```python
from build123d import *

# Parameters (mm, degrees)
BOSS_EXTRUDE1_DEPTH     = 5
BOSS_EXTRUDE2_DEPTH     = 27.5
BOSS_EXTRUDE3_DEPTH     = 10
CUT_EXTRUDE2_DEPTH      = 51.717354111
CUT_EXTRUDE2_DEPTH_BACK = 51.717354111
SKETCH5_3_W             = 6.5
SKETCH5_3_H             = 2
SKETCH5_3_W_2           = 20
BOSS_EXTRUDE4_DEPTH     = 2.75
CUT_EXTRUDE3_DEPTH      = 54.359629019
CUT_EXTRUDE3_DEPTH_BACK = 24
M4_CLEARANCE_HOLE1_D    = 4.5


with BuildPart() as part:
    # Sketch1 → Boss-Extrude1 (new body)
    with BuildSketch(Plane(origin=(0, 0, 0), x_dir=(1, 0, 0), z_dir=(0, 1, 0))):
        with BuildLine():
            Line((-36.5, 15), (36.5, 15))
            ThreePointArc((36.5, 15), (40.035533906, 13.535533906), (41.5, 10))
            Line((41.5, 10), (41.5, -10))
            ThreePointArc((41.5, -10), (40.035533906, -13.535533906), (36.5, -15))
            Line((36.5, -15), (-36.5, -15))
            ThreePointArc((-36.5, -15), (-40.035533906, -13.535533906), (-41.5, -10))
            Line((-41.5, -10), (-41.5, 10))
            ThreePointArc((-41.5, 10), (-40.035533906, 13.535533906), (-36.5, 15))
        make_face()
        with BuildLine():
            Line((-31.5, 7.5), (-31.5, -7.5))
            ThreePointArc((-31.5, -7.5), (-34.5, -10.5), (-37.5, -7.5))
            Line((-37.5, -7.5), (-37.5, 7.5))
            ThreePointArc((-37.5, 7.5), (-34.5, 10.5), (-31.5, 7.5))
        make_face(mode=Mode.SUBTRACT)
        with BuildLine():
            Line((31.5, 7.5), (31.5, -7.5))
            ThreePointArc((31.5, -7.5), (34.5, -10.5), (37.5, -7.5))
            Line((37.5, -7.5), (37.5, 7.5))
            ThreePointArc((37.5, 7.5), (34.5, 10.5), (31.5, 7.5))
        make_face(mode=Mode.SUBTRACT)
    extrude(amount=-BOSS_EXTRUDE1_DEPTH)

    # Sketch2 → Boss-Extrude2 (add, symmetric)
    with BuildSketch(Plane(origin=(0, 0, 0), x_dir=(0, 0, -1), z_dir=(1, 0, 0))):
        with BuildLine():
            Line((-15, 0), (0, 0))
            Line((0, 0), (0, 18))
            Line((0, 18), (-2.75, 18))
            add(Edge.make_bspline(
                [(-15, 0), (-3.342305564, 4.287493928), (-2.75, 18)],
                knots=[0, 0, 0, 1, 1, 1], degree=2))
        make_face()
        with BuildLine():
            Line((0, 18), (0, 0))
            Line((0, 0), (15, 0))
            add(Edge.make_bspline(
                [(15, 0), (3.342305564, 4.287493928), (2.75, 18)],
                knots=[0, 0, 0, 1, 1, 1], degree=2))
            Line((2.75, 18), (0, 18))
        make_face()
    extrude(amount=BOSS_EXTRUDE2_DEPTH, both=True)

    # Sketch2<3> → Boss-Extrude3 (add, symmetric)
    with BuildSketch(Plane(origin=(0, 0, 0), x_dir=(0, 0, -1), z_dir=(1, 0, 0))):
        with BuildLine():
            Line((-15, 0), (-15, 25))
            Line((-15, 25), (-8, 25))
            Line((-8, 25), (-2.75, 23))
            Line((-2.75, 23), (-2.75, 18))
            add(Edge.make_bspline(
                [(-15, 0), (-3.342305564, 4.287493928), (-2.75, 18)],
                knots=[0, 0, 0, 1, 1, 1], degree=2))
        make_face()
        with BuildLine():
            add(Edge.make_bspline(
                [(15, 0), (3.342305564, 4.287493928), (2.75, 18)],
                knots=[0, 0, 0, 1, 1, 1], degree=2))
            Line((2.75, 18), (2.75, 23))
            Line((2.75, 23), (8, 25))
            Line((8, 25), (15, 25))
            Line((15, 25), (15, 0))
        make_face()
    extrude(amount=BOSS_EXTRUDE3_DEPTH, both=True)

    # Sketch5 → Cut-Extrude2 (cut, two sides: drawn at the far end of the back side and taken through both)
    with BuildSketch(Plane.XY.offset(-CUT_EXTRUDE2_DEPTH_BACK)):
        Polygon((-27.5, 18), (-27.5, 0), (-21.5, 18), align=None)
        Polygon((21.5, 18), (27.5, 0), (27.5, 18), align=None)
    extrude(amount=CUT_EXTRUDE2_DEPTH + CUT_EXTRUDE2_DEPTH_BACK, mode=Mode.SUBTRACT)

    # Sketch5<3> → Boss-Extrude4 (add, symmetric)
    with BuildSketch(Plane.XY):
        with Locations((13.25, 19)):
            Rectangle(SKETCH5_3_W, SKETCH5_3_H)
        with Locations((-13.25, 19)):
            Rectangle(SKETCH5_3_W, SKETCH5_3_H)
        with Locations((0, 19)):
            Rectangle(SKETCH5_3_W_2, SKETCH5_3_H)
    extrude(amount=BOSS_EXTRUDE4_DEPTH, both=True)

    # Sketch6 → Cut-Extrude3 (cut, two sides: drawn at the far end of the back side and taken through both)
    with BuildSketch(Plane.XZ.offset(5).offset(-CUT_EXTRUDE3_DEPTH_BACK)):
        Polygon((16, 2.25), (10, 2.25), (-10, 2.25), (-16, 2.25), (-16, -2.25), (-10, -2.25), (10, -2.25), (16, -2.25), align=None)
    extrude(amount=CUT_EXTRUDE3_DEPTH + CUT_EXTRUDE3_DEPTH_BACK, mode=Mode.SUBTRACT)

    # M4 Clearance Hole1 (through all)
    with Locations(Plane(origin=(0, 20, 0), x_dir=(1, 0, 0), z_dir=(0, 1, 0))):
        with Locations((0, 0)):
            Hole(M4_CLEARANCE_HOLE1_D / 2)


solid = part.part
```
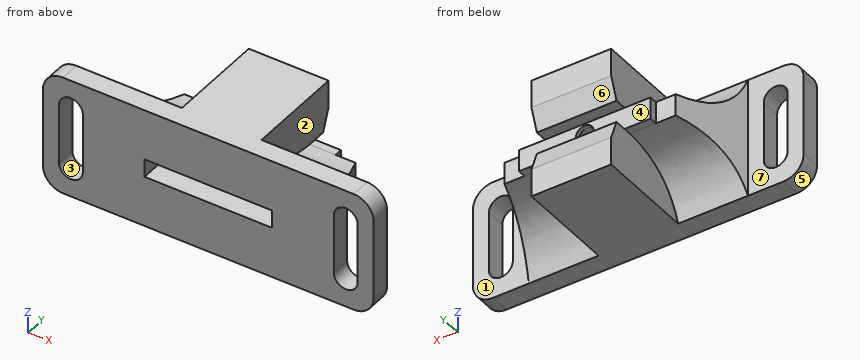
For this review, take the finished solid that the model builds, in its own axes (mm). Face numbers are marked on the shaded views. A direction names the side the tool comes from. Coordinates: 2 decimals unless noted, no trailing zeros. Write each loop counter-clockwise with the first axis right and the second up, starting at its lowest first coordinate (ties: lowest second). Pieces come first, ordered by that corner, then holes. Notation, with made-up numbers: (16, -36.75) - (26, -36.75) arc R29 cw to (26, -11.75) - close; hole circle Ø4 at (3, 49). An arc over 180 degrees is marked (long way). Answer in a Markdown table with one row per item. Add a question column.
Q1. We need section C-C, the plane z = 6.5. Count the separate pieces of the cut face and the enclosed holes in it, and give its area (3 significant figures).
Q2. We need section B-B, the plane z = 0. State the section outline as (x, y) points, and give its area (4 significant figures).
Q3. Draft analysis for pull direction Z (two halves, no side actions). For the marked faces 5, 6 and 7, state which applies: +Z half, -Z half, draft (parallel to the pull), parting line (faces both ways), or undercut.
Q4. Tool access review of the marked faces 1, 2, 3 and 4: name each direction out of +Z, -Z, +X, -X, +Y, -Y from which nothing blocks a thin tool from reaching the whole face with its end or side.
Q5. For P1, Ø1, axis at y = 17, z = -2, coming from the -X side; P2, Ø4, axis at x = 36.5, z = -2.5, coming from the +Y side; P3, Ø1, axis at y = 4.5, z = 11, coming from the -X side, all flat-tipped, find the tip position at first contact; note any pin that passes through.
Q6. We need section A-A, the plane x = -34.5. State the section outline as (y, z) points.
Q7. For probe 1 along X at (y, z) = (-1, 0); probe 2 along Z at (x, y) = (0, 19.45); probe 3 along Z at (x, y) = (-0.5, 22.5), list the stretches that pass through material, from the lowest coordinate up.
Answer list:
| question | item | result |
|---|---|---|
| 1 | separate pieces | 3 |
| 1 | enclosed holes | 0 |
| 1 | area | 1,040 mm2 |
| 2 | outline | (-41.5, -5) - (-37.5, -5) - (-37.5, 0) - (-41.5, 0) - close; (-31.5, -5) - (-16, -5) - (-16, 19) - (-2.25, 19) - (-2.25, 20) - (-16.5, 20) - (-16.5, 18) - (-21.5, 18) - (-27.5, 0) - (-31.5, 0) - close; (2.25, 19) - (16, 19) - (16, -5) - (31.5, -5) - (31.5, 0) - (27.5, 0) - (21.5, 18) - (16.5, 18) - (16.5, 20) - (2.25, 20) - close; (37.5, -5) - (41.5, -5) - (41.5, 0) - (37.5, 0) - close |
| 2 | area | 530.5 mm2 |
| 3 | face 5 | -Z half |
| 3 | face 6 | undercut |
| 3 | face 7 | draft |
| 4 | face 1 | +Z, -Z, +X, +Y |
| 4 | face 2 | +Z, +X, +Y |
| 4 | face 3 | +Y, -Y |
| 4 | face 4 | +X, -X, +Y |
| 5 | P1 | stops at x = -22 |
| 5 | P2 | stops at y = 0 |
| 5 | P3 | stops at x = -10 |
| 6 | outline | (-5, -15) - (0, -15) - (0, -10.5) - (-5, -10.5) - close; (-5, 10.5) - (0, 10.5) - (0, 15) - (-5, 15) - close |
| 7 | probe 1 | x = -41.5 to -37.5, -31.5 to -16, 16 to 31.5, 37.5 to 41.5 |
| 7 | probe 2 | z = -15 to -2.25, 2.25 to 15 |
| 7 | probe 3 | z = -15 to -2.75, 2.75 to 15 |
